Verification items for the finished model (mm, model axes). A direction names the side the tool comes from. Give positions to 0.01 mm unless a question says otherwise; leave off trailing zeros. Order: outer loops, then holes, each group sorted by start corner. A loop starts at its lowest first (then second) coordinate and runs counter-clockwise, first axis right, second up. Notation, with made-up numbers: M 52.25,43.5 L 56.25,43.5 A30 ccw 56.25,65.5 Z; hole C 81.5,8 d2. An arc over 180 degrees is marked long. Answer as a JSON object with one key per item and string values.
```python
from build123d import *

# Parameters (mm, degrees)
SKETCH_1_W                     = 210
SKETCH_1_H                     = 50
EXTRUDE_1_DEPTH                = 5
SKETCH_3_R                     = 2.25
CUT_EXTRUDE_1_DEPTH            = 5
SKETCH_4_W                     = 210
SKETCH_4_H                     = 5
EXTRUDE_2_DEPTH                = 61
CUT_EXTRUDE_2_REACH            = 227.734
SKETCH_6_W                     = 60
SKETCH_6_H                     = 5
FILLET_1_R                     = 10
CUT_EXTRUDE_3_REACH            = 227.734
SKETCH_7_W                     = 88
SKETCH_7_H                     = 5
FILLET_2_R                     = 10
FILLET_6_R                     = 3
SKETCH_11_R                    = 2.25
CUT_EXTRUDE_4_DEPTH            = 225.67977212
SPLIT_BODIES_2_SURFACE_1_BACK  = 429.084
SPLIT_BODIES_2_SURFACE_1_DEPTH = 858.168
FILLET_8_R                     = 5
FILLET_9_R                     = 3


# Some blends are built 0.0001 mm under size
with BuildPart() as part:
    # 草图1 → 凸台-拉伸1 (new body)
    with BuildSketch(Plane.XY):
        with Locations((105, 25)):
            Rectangle(SKETCH_1_W, SKETCH_1_H)
    extrude_1 = extrude(amount=EXTRUDE_1_DEPTH)

    # 草图3 → 切除-拉伸1 (cut)
    with BuildSketch(Plane.XY.offset(5)):
        with Locations((157.25, 25)):
            Circle(SKETCH_3_R)
        with Locations((187.25, 25)):
            Circle(SKETCH_3_R)
        with Locations(Location((22.75, 25, 0), (0, 0, 180))):
            Circle(SKETCH_3_R)
        with Locations(Location((52.75, 25, 0), (0, 0, 180))):
            Circle(SKETCH_3_R)
    cut_extrude_1 = extrude(amount=-CUT_EXTRUDE_1_DEPTH, mode=Mode.SUBTRACT)

    # 草图4 → 凸台-拉伸2 (add)
    with BuildSketch(Plane.XY.offset(5)):
        with Locations((105, 2.5)):
            Rectangle(SKETCH_4_W, SKETCH_4_H)
    extrude_2 = extrude(amount=EXTRUDE_2_DEPTH)

    # 草图6 → 切除-拉伸2 (cut, up to next)
    with BuildSketch(Plane.XY.offset(66), mode=Mode.PRIVATE) as cut_extrude_2_sk1:
        with Locations((180, 2.5)):
            Rectangle(SKETCH_6_W, SKETCH_6_H)
    cut_extrude_2_tool1 = extrude(cut_extrude_2_sk1.sketch, amount=-CUT_EXTRUDE_2_REACH, mode=Mode.PRIVATE) & part.part
    cut_extrude_2 = cut_extrude_2_tool1.solids().sort_by_distance((180, 2.5, 66))[0]
    add(cut_extrude_2, mode=Mode.SUBTRACT)

    # 圆角1
    # the kernel refuses this fillet: 10 mm, written as the material it adds along each edge
    with BuildSketch(Plane(origin=(150, 5, 0), x_dir=(0, -1, 0), z_dir=(0, 0, 1))) as fillet_1_piece_1:
        with BuildLine():
            CenterArc((10, 8.660254038), FILLET_1_R, 180, 60)
            Line((0, 8.660254038), (0, 0))
            Line((0, 0), (5, 0))
        make_face()
    extrude(amount=5)

    # 草图7 → 切除-拉伸3 (cut, up to next)
    with BuildSketch(Plane.XY.offset(66), mode=Mode.PRIVATE) as cut_extrude_3_sk1:
        with Locations((44, 2.5)):
            Rectangle(SKETCH_7_W, SKETCH_7_H)
    cut_extrude_3_tool1 = extrude(cut_extrude_3_sk1.sketch, amount=-CUT_EXTRUDE_3_REACH, mode=Mode.PRIVATE) & part.part
    cut_extrude_3 = cut_extrude_3_tool1.solids().sort_by_distance((44, 2.5, 66))[0]
    add(cut_extrude_3, mode=Mode.SUBTRACT)

    # 圆角2
    # the kernel refuses this fillet: 10 mm, written as the material it adds along each edge
    with BuildSketch(Plane(origin=(88, 5, 0), x_dir=(0, -1, 0), z_dir=(0, 0, 1))) as fillet_2_piece_1:
        with BuildLine():
            CenterArc((10, -8.660254038), FILLET_2_R, 120, 60)
            Line((0, -8.660254038), (0, 0))
            Line((0, 0), (5, 0))
        make_face()
    extrude(amount=5)

    # 圆角6
    # the kernel refuses this fillet: 3 mm, written as the material it adds along each edge
    with BuildSketch(Plane(origin=(150, 5, 5), x_dir=(1, 0, 0), z_dir=(0, -1, 0))) as fillet_6_piece_1_section:
        with BuildLine():
            CenterArc((FILLET_6_R, FILLET_6_R), FILLET_6_R, 180, 90)
            Line((0, FILLET_6_R), (0, 0))
            Line((0, 0), (FILLET_6_R, 0))
        make_face()
    fillet_6_piece_1 = extrude(amount=5, mode=Mode.PRIVATE)
    fillet_6_piece_1 = fillet_6_piece_1 - Plane(origin=(158.660254038, -5, 5.756133445), x_dir=(0, -1, 0), z_dir=(0, 0, -1)) * Cylinder(10, 22, mode=Mode.PRIVATE)
    add(fillet_6_piece_1)
    with BuildSketch(Plane(origin=(88, 5, 5), x_dir=(-1, 0, 0), z_dir=(0, -1, 0))) as fillet_6_piece_2_section:
        with BuildLine():
            CenterArc((FILLET_6_R, -FILLET_6_R), FILLET_6_R, 90, 90)
            Line((0, -FILLET_6_R), (0, 0))
            Line((0, 0), (FILLET_6_R, 0))
        make_face()
    fillet_6_piece_2 = extrude(amount=5, mode=Mode.PRIVATE)
    fillet_6_piece_2 = fillet_6_piece_2 - Plane(origin=(79.339745962, -5, 5.756136784), x_dir=(0, -1, 0), z_dir=(0, 0, -1)) * Cylinder(10, 22, mode=Mode.PRIVATE)
    add(fillet_6_piece_2)

    # 草图11 → 切除-拉伸4 (cut, through all)
    with BuildSketch(Plane(origin=(0, 5, 0), x_dir=(1, 0, 0), z_dir=(0, 1, 0))):
        with Locations(Location((98.991167509, -29.5, 0), (0, 0, 180))):
            Circle(SKETCH_11_R)
        with Locations(Location((138.991167509, -29.5, 0), (0, 0, 180))):
            Circle(SKETCH_11_R)
        with Locations(Location((98.991167509, -41.5, 0), (0, 0, 180))):
            Circle(SKETCH_11_R)
        with Locations(Location((138.991167509, -41.5, 0), (0, 0, 180))):
            Circle(SKETCH_11_R)
    cut_extrude_4 = extrude(amount=-CUT_EXTRUDE_4_DEPTH, mode=Mode.SUBTRACT)

    # 镜向16: 凸台-拉伸1, 切除-拉伸1, 凸台-拉伸2, 切除-拉伸2, 切除-拉伸3, 切除-拉伸4 across plane
    add(extrude_1.mirror(Plane(origin=(210, 0, 5), x_dir=(0, 0, 1), z_dir=(-1, 0, 0))))
    add(cut_extrude_1.mirror(Plane(origin=(210, 0, 5), x_dir=(0, 0, 1), z_dir=(-1, 0, 0))), mode=Mode.SUBTRACT)
    add(extrude_2.mirror(Plane(origin=(210, 0, 5), x_dir=(0, 0, 1), z_dir=(-1, 0, 0))))
    add(cut_extrude_2.mirror(Plane(origin=(210, 0, 5), x_dir=(0, 0, 1), z_dir=(-1, 0, 0))), mode=Mode.SUBTRACT)
    add(cut_extrude_3.mirror(Plane(origin=(210, 0, 5), x_dir=(0, 0, 1), z_dir=(-1, 0, 0))), mode=Mode.SUBTRACT)
    add(cut_extrude_4.mirror(Plane(origin=(210, 0, 5), x_dir=(0, 0, 1), z_dir=(-1, 0, 0))), mode=Mode.SUBTRACT)

    # Split Bodies 2: cut with a surface, the side it looks to stays
    # Split Bodies 2 surface: a surface, the sketch's curves swept straight by 858.168 mm
    with BuildLine(Plane.XY.offset(5).offset(-SPLIT_BODIES_2_SURFACE_1_BACK), mode=Mode.PRIVATE) as split_bodies_2_surface_1_path:
        Line((210, 50), (210, 0))
    split_bodies_2_surface_1 = Shell.extrude(split_bodies_2_surface_1_path.wire(), (0 * SPLIT_BODIES_2_SURFACE_1_DEPTH, 0 * SPLIT_BODIES_2_SURFACE_1_DEPTH, 1 * SPLIT_BODIES_2_SURFACE_1_DEPTH))
    split(bisect_by=split_bodies_2_surface_1, keep=Keep.TOP)

    # 圆角8
    fillet_8_edges = [part.edges().sort_by_distance(p)[0] for p in [
        (332, 5, 2.5),
        (270, 5, 2.5),
    ]]
    fillet(fillet_8_edges, radius=FILLET_8_R - 0.0001)  # a hair under: the kernel refuses the full size

    # 圆角9
    fillet_9_edges = [part.edges().sort_by_distance(p)[0] for p in [
        (332, 2.50005, 5),
        (270, 2.50005, 5),
    ]]
    fillet(fillet_9_edges, radius=FILLET_9_R)


solid = part.part
```
Q1. Gauge pin test, flat ends, axial feed: pin 1 Ø2.5 at (x, z) = (281.01, 29.5) entering from +Y; pin 2 Ø1.5 at (y, z) = (2.5, 38) entering from -X; pin 3 Ø4 at (y, z) = (3, 43.5) entering from +X; pin 4 Ø18.5 at (x, z) = (311, 49) entering from +Y. Record the tip position at first contact, or that the pin passes through.
Resolved:
{"pin 1": "passes through", "pin 2": "stops at x = 270", "pin 3": "stops at x = 332", "pin 4": "stops at y = 5"}
Q2. Section check C-C on y = 10.5. Record the cut outline in (x, z), then the cut area to 3 significant figures.
Resolved:
{"outline": "M 210,0 L 420,0 L 420,5 L 210,5 Z", "area": "1,050 mm²"}
Q3. Material ranges on L1, parallel to Y at x = 262.75, z = 2.2; L2, parallel to Z at x = 370, y = 15, recorded low to high.
Resolved:
{"L1": "y = 5 to 22.75, 27.25 to 50", "L2": "z = 0 to 5"}
Q4. Section check B-B on x = 293.5. Record the cut outline in (y, z), then the cut area to 3 significant figures.
Resolved:
{"outline": "M 0,0 L 50,0 L 50,5 L 5,5 L 5,66 L 0,66 Z", "area": "555 mm²"}
Q5. Tool access check on faces 5 (the face through (301, 5, 35)), 6 (the face through (301, 0, 33)), 7 (the face through (379, 5, 3)), 8 (the face through (270, 2, 33)). Record the directions out of +Z, -Z, +X, -X, +Y, -Y that give a thin tool (end or side, any length) a straight path to the whole face; none if there is none.
Resolved:
{"face 5": "+Z, +X, -X, +Y", "face 6": "+Z, -Z, +X, -X, -Y", "face 7": "+Z, -Z, +X, -Y", "face 8": "+Z, -X, +Y, -Y"}
Q6. Section check A-A on x = 397.25. Record the cut outline in (y, z), then the cut area to 4 significant figures.
Resolved:
{"outline": "M 5,0 L 22.75,0 L 22.75,5 L 5,5 Z; M 27.25,0 L 50,0 L 50,5 L 27.25,5 Z", "area": "202.5 mm²"}
Q7. Section check D-D on z = 46. Record the cut outline in (x, y), then the cut area to 3 significant figures.
Resolved:
{"outline": "M 270,0 L 332,0 L 332,5 L 270,5 Z", "area": "310 mm²"}
Q8. Release check for a two-part mould opening along X. For faces 1 (the face through (278.76, 2.54, 29.6)), 2 (the face through (301, 3, 66)), 3 (the face through (420, 27, 2)), 4 (the face through (365, 25, 3)) record: +X half, -X half, draft (parallel to the pull), parting line (faces both ways), or undercut.
Resolved:
{"face 1": "undercut", "face 2": "draft", "face 3": "+X half", "face 4": "undercut"}
